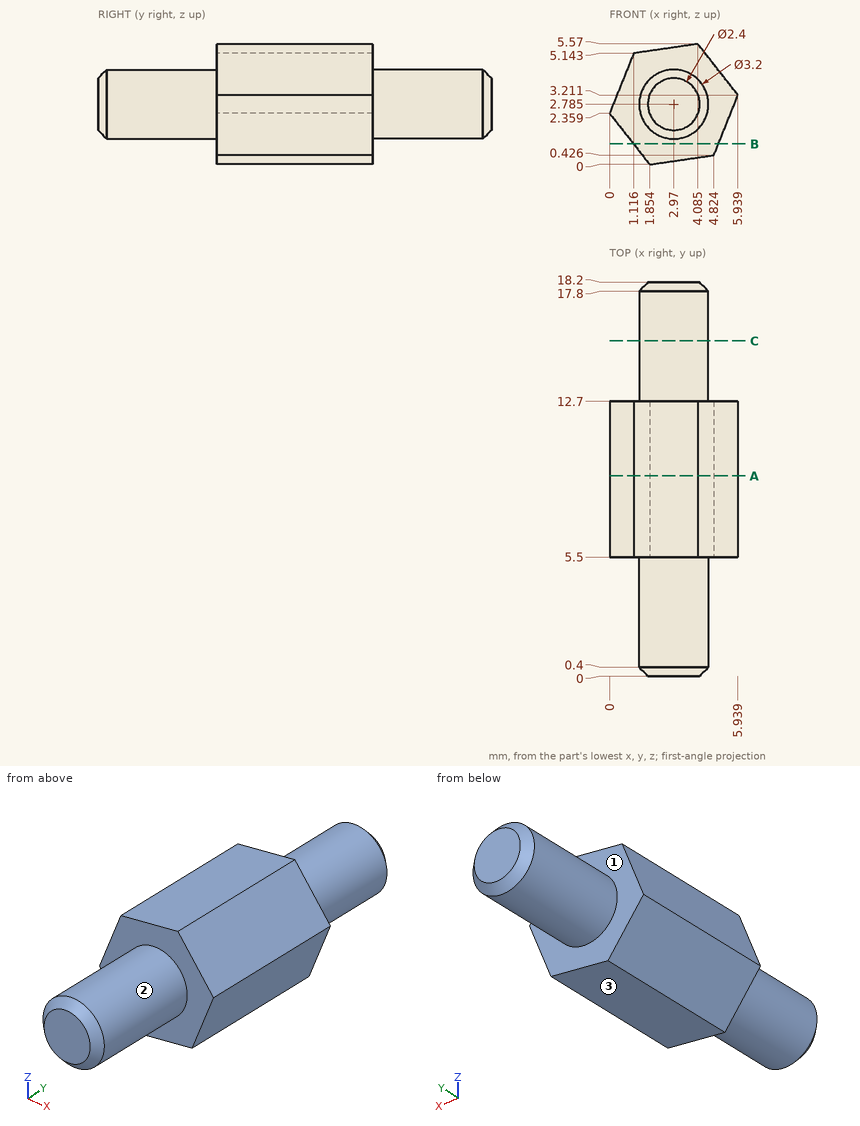
The figure shows three views and two pictorial views of one solid part (mm, origin at its lowest corner). Answer the questions. A direction names the side the tool comes from. Round coordinates to 2 decimals unless told otherwise and drop trailing zeros. Write each loop counter-clockwise with the first axis right and the second up, starting at its lowest first coordinate (ties: lowest second). Pieces come first, ordered by that corner, then holes. Notation, with made-up numbers: (27.5, 26.25) - (67.5, 26.25) arc R31 ccw to (67.5, 51.25) - close; hole circle Ø11 at (16, 87). An arc over 180 degrees is marked (long way). Answer in a Markdown table with one row per item. Add a question column.
1. Given pin 1 (3 mm diameter, centred on x = 5, y = 3.5, fed in from +Z) (1 decimal); pin 2 (1 mm diameter, centred on x = 5, z = 4, fed in from -Y); pin 3 (1 mm diameter, centred on x = 1.5, y = 16, fed in from +Z); pin 4 (3 mm diameter, centred on x = 3.5, z = 2, fed in from -Y), each flat-ended and moving along its own axis, determine where each tip first touches the part or whether it passes through.
2. A cutting plane is placed at B-B, the plane z = 0.95. Determine the outline of the cut face in (x, y).
3. A cutting plane is placed at A-A, the plane y = 9.25. Determine the outline of the cut face in (x, z) (1 decimal), and give its area (3 significant figures).
4. Find the intervals of material crossed by line 1 along Y through (x, z) = (1.6, 5); line 2 along Y through (x, z) = (2, 3.5) (1 decimal); line 3 along X through (y, z) = (1.75, 1.5) (1 decimal), in increasing order. Write a range as from..to.
5. For the marked faces 1, 2 and 3, determine the directions among +Z, -Z, +X, -X, +Y, -Y from which every point of the face is accessible in a straight line to the end or side of a thin tool.
6. A cutting plane is placed at C-C, the plane y = 15.5. Determine the outline of the cut face in (x, z) (1 decimal).
Worked out:
| question | item | result |
|---|---|---|
| 1 | pin 1 | z = 4.3 |
| 1 | pin 2 | y = 5.5 |
| 1 | pin 3 | z = 4.06 |
| 1 | pin 4 | y = 0 |
| 2 | outline | (1.11, 5.5) - (5.03, 5.5) - (5.03, 12.7) - (1.11, 12.7) - close |
| 3 | outline | (0, 2.4) - (1.9, 0) - (4.8, 0.4) - (5.9, 3.2) - (4.1, 5.6) - (1.1, 5.1) - close |
| 3 | area | 23.4 mm^2 |
| 4 | line 1 | 5.5..12.7 |
| 4 | line 2 | 0..18.2 |
| 4 | line 3 | 2..3.9 |
| 5 | face 1 | +Y |
| 5 | face 2 | -Y |
| 5 | face 3 | -Z, +X, +Y, -Y |
| 6 | outline | circle Ø3.2 at (3, 2.8) |
